Design review of the part built by this model. Coordinates are the model's own, in mm. Face numbers are marked on the shaded views. A direction names the side the tool comes from. Give positions to 0.01 mm unless a question says otherwise; leave off trailing zeros. Loops run counter-clockwise (first coordinate to the right, second up) from the corner with the lowest first, then second, coordinate; pieces in that order, holes last. Notation, with made-up numbers: M 30.25,-37.5 L 84.25,-37.5 A19 ccw 84.25,-27.5 Z; hole C -40,18.5 d2. An arc over 180 degrees is marked long. Use a Markdown table: item, result. Add a question column.
(1) Add section A-A, the plane x = 0. Give the boundary of the cut face in (y, z) (3 decimals), then the cut area to 3 significant figures.
(2) Draft analysis for pull direction X (two halves, no side actions). For the marked faces 4, 5 and 6, state which applies: pulls with the +X half, pulls with the -X half, needs draft (parallel to the pull), parting line crosses it, or undercut.
(3) Add section B-B, the plane y = -5.5. Give the boundary of the cut face in (x, z).
(4) Add section D-D, the plane x = 12.7. Give the boundary of the cut face in (y, z) (3 decimals).
(5) Insertion check: pin 1 Ø7.5 at (x, y) = (-12.7, 3.175) entering from +Z (3 decimals); pin 2 Ø8 at (x, z) = (-1.5, 20.5) entering from +Y (3 decimals); pin 3 Ø3 at (x, z) = (0, 17.653) entering from -Y. Each pin has a flat end and moves straight along its axis. Give the tip position at first contact, or say it passes through.
(6) For probe 1 along Z at (x, y) = (0, -4.5); probe 2 along Y at (x, z) = (1.5, 15.5) (3 decimals); probe 3 along Z at (x, y) = (-10, 3.5) (3 decimals), list the stretches that pass through material, from the lowest coordinate up.
(7) Add section C-C, the plane y = 1.5. Give the boundary of the cut face in (x, z) (3 decimals).
(8) For the marked faces 1, 2 and 3, list the 3-axis set-ups (+Z, -Z, +X, -X, +Y, -Y) from which the entire face can be reached by the end or side of a thin tool; tool diameter is ignored.
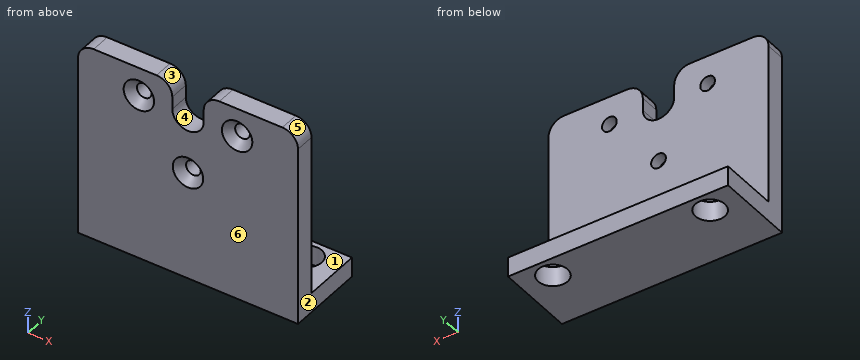
```python
from build123d import *

# Parameters (mm, degrees)
SKETCH1_W           = 35.56
SKETCH1_H           = 12.7
SKETCH1_R           = 2.38125
BOSS_EXTRUDE1_DEPTH = 3.175
SKETCH7_W           = 35.56
SKETCH7_H           = 3.175
BOSS_EXTRUDE3_DEPTH = 28.575
SKETCH11_R          = 1.190625
CUT_EXTRUDE1_DEPTH  = 13.7
FILLET1_R           = 2.54
CHAMFER2_SIZE       = 1.27


with BuildPart() as part:
    # Sketch1 → Boss-Extrude1 (new body)
    with BuildSketch(Plane.XY):
        Rectangle(SKETCH1_W, SKETCH1_H)
        with Locations((-12.7, 3.175)):
            Circle(SKETCH1_R, mode=Mode.SUBTRACT)
        with Locations((12.7, 3.175)):
            Circle(SKETCH1_R, mode=Mode.SUBTRACT)
    extrude(amount=BOSS_EXTRUDE1_DEPTH)

    # Sketch7 → Boss-Extrude3 (add)
    with BuildSketch(Plane.XY.offset(3.175)):
        with Locations((0, -4.7625)):
            Rectangle(SKETCH7_W, SKETCH7_H)
    extrude(amount=BOSS_EXTRUDE3_DEPTH)

    # Sketch11 → Cut-Extrude1 (cut, through all)
    with BuildSketch(Plane.XZ.offset(6.35)):
        with Locations((-7.9375, 27.178)):
            Circle(SKETCH11_R)
        with Locations((7.9375, 27.178)):
            Circle(SKETCH11_R)
        with Locations((0, 17.653)):
            Circle(SKETCH11_R)
        with BuildLine():
            Line((-2.54, 48.261780908), (2.54, 48.261780908))
            Line((2.54, 48.261780908), (2.54, 27.178))
            ThreePointArc((2.54, 27.178), (0, 24.638), (-2.54, 27.178))
            Line((-2.54, 27.178), (-2.54, 48.261780908))
        make_face()
    extrude(amount=-CUT_EXTRUDE1_DEPTH, mode=Mode.SUBTRACT)

    # Fillet1
    fillet1_edges = [part.edges().sort_by_distance(p)[0] for p in [
        (-17.78, -4.7625, 31.75),
        (17.78, -4.7625, 31.75),
        (2.54, -4.7625, 31.75),
        (-2.54, -4.7625, 31.75),
    ]]
    fillet(fillet1_edges, radius=FILLET1_R)

    # Chamfer2
    chamfer2_edges = [part.edges().sort_by_distance(p)[0] for p in [
        (-9.128125, -6.35, 27.178),
        (6.746875, -6.35, 27.178),
        (-1.190625, -6.35, 17.653),
    ]]
    chamfer(chamfer2_edges, length=CHAMFER2_SIZE)


solid = part.part
```
Established:
| question | item | result |
|---|---|---|
| 1 | outline | M -6.35,0 L 6.35,0 L 6.35,3.175 L -3.175,3.175 L -3.175,16.462 L -5.08,16.462 L -6.35,15.192 Z; M -6.35,20.114 L -5.08,18.844 L -3.175,18.844 L -3.175,24.638 L -6.35,24.638 Z |
| 1 | area | 99.3 mm^2 |
| 2 | face 4 | undercut |
| 2 | face 5 | pulls with the +X half |
| 2 | face 6 | needs draft |
| 3 | outline | M -17.78,0 L 17.78,0 L 17.78,29.21 A2.54 ccw 15.24,31.75 L 5.08,31.75 A2.54 ccw 2.54,29.21 L 2.54,27.18 A2.54 cw -2.54,27.18 L -2.54,29.21 A2.54 ccw -5.08,31.75 L -15.24,31.75 A2.54 ccw -17.78,29.21 Z; hole C -7.94,27.18 d3.22; hole C 0,17.65 d3.22; hole C 7.94,27.18 d3.22 |
| 4 | outline | M -6.35,0 L 0.794,0 L 0.794,3.175 L -3.175,3.175 L -3.175,31.75 L -6.35,31.75 Z; M 5.556,0 L 6.35,0 L 6.35,3.175 L 5.556,3.175 Z |
| 5 | pin 1 | z = 3.175 |
| 5 | pin 2 | y = -3.175 |
| 5 | pin 3 | y = -5.39 |
| 6 | probe 1 | 0 to 16.46, 18.84 to 24.64 |
| 6 | probe 2 | -6.35 to -3.175 |
| 6 | probe 3 | 0 to 3.175 |
| 7 | outline | M -17.78,0 L -14.393,0 L -14.393,3.175 L -17.78,3.175 Z; M -11.007,0 L 11.007,0 L 11.007,3.175 L -11.007,3.175 Z; M 14.393,0 L 17.78,0 L 17.78,3.175 L 14.393,3.175 Z |
| 8 | face 1 | +Z, +X, -X, +Y |
| 8 | face 2 | +Z, -Z, +X, +Y, -Y |
| 8 | face 3 | +Z, +Y, -Y |
